Check sheet for the drawn part. Datum: minimum x, y, z corner. Units: mm. A direction names the side the tool comes from. Round coordinates to 2 decimals unless told otherwise and drop trailing zeros. Loops run counter-clockwise (first coordinate to the right, second up) from the corner with the lowest first, then second, coordinate; pieces in that order, holes last. Notation, with made-up numbers: (67.25, 14) - (125.25, 14) arc R17 ccw to (125.25, 30) - close; hole circle Ø11 at (50, 22.5). An arc over 180 degrees is marked (long way). Use CSV: the item, a comma, the result in double quotes.
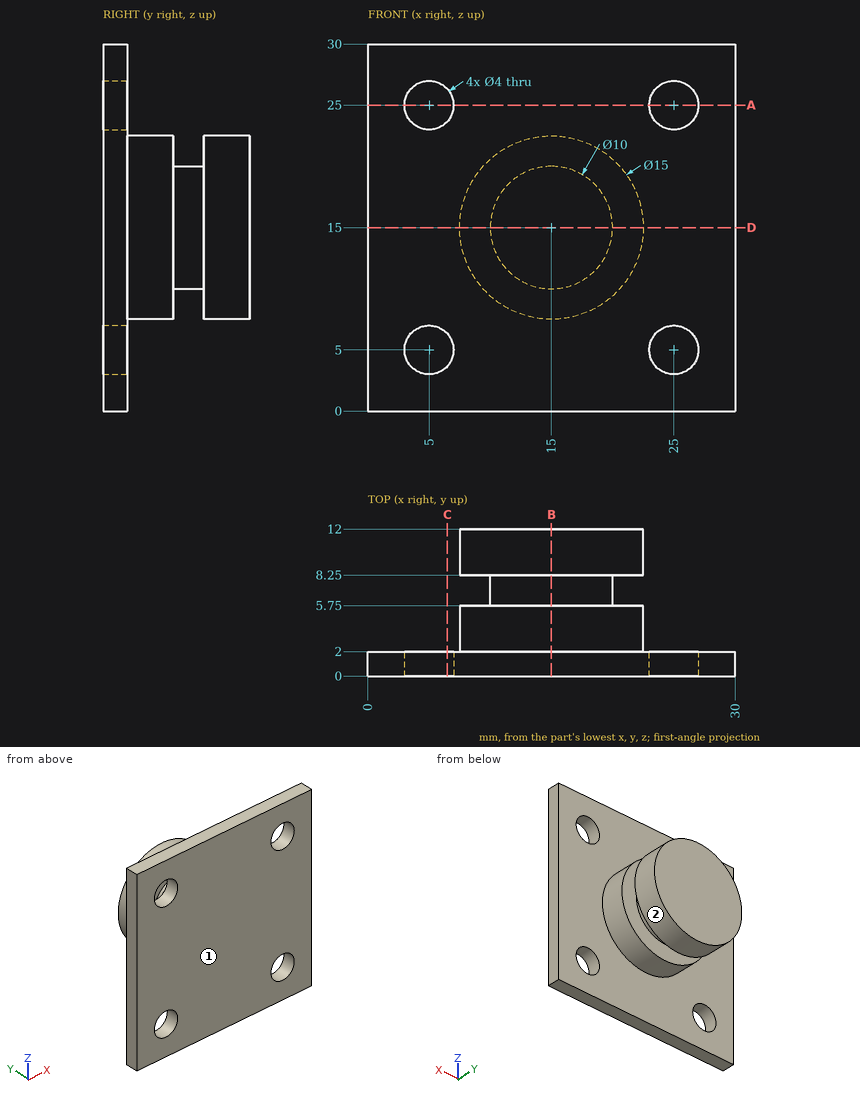
1) Cross-section at A-A, the plane z = 25. Record the cut outline in (x, y).
Returned:
outline,"(0, 0) - (3, 0) - (3, 2) - (0, 2) - close; (7, 0) - (23, 0) - (23, 2) - (7, 2) - close; (27, 0) - (30, 0) - (30, 2) - (27, 2) - close"
2) Cross-section at D-D, the plane z = 15. Record the cut outline in (x, y).
Returned:
outline,"(0, 0) - (30, 0) - (30, 2) - (22.5, 2) - (22.5, 5.75) - (20, 5.75) - (20, 8.25) - (22.5, 8.25) - (22.5, 12) - (7.5, 12) - (7.5, 8.25) - (10, 8.25) - (10, 5.75) - (7.5, 5.75) - (7.5, 2) - (0, 2) - close"
3) Thickness scan on probe 1 along X at (y, z) = (0.7, 5); probe 2 along Y at (x, z) = (14.25, 9.75). Record the ranges inside material, lowest first. Write a range as [from, to].
Returned:
probe 1,"x = [0, 3], [7, 23], [27, 30]"
probe 2,"y = [0, 5.75], [8.25, 12]"
4) Access from +Z, -Z, +X, -X, +Y, -Y to the whole of each face (thin tool, end or side, straight path). Record for the marked faces 1 and 2.
Returned:
face 1,"+Z, -Z, +X, -X, -Y"
face 2,"+Y"
5) Cross-section at B-B, the plane x = 15. Record the cut outline in (y, z).
Returned:
outline,"(0, 0) - (2, 0) - (2, 7.5) - (5.75, 7.5) - (5.75, 10) - (8.25, 10) - (8.25, 7.5) - (12, 7.5) - (12, 22.5) - (8.25, 22.5) - (8.25, 20) - (5.75, 20) - (5.75, 22.5) - (2, 22.5) - (2, 30) - (0, 30) - close"
6) Cross-section at C-C, the plane x = 6.5. Record the cut outline in (y, z), then the cut area to 3 significant figures.
Returned:
outline,"(0, 0) - (2, 0) - (2, 3.68) - (0, 3.68) - close; (0, 6.32) - (2, 6.32) - (2, 23.68) - (0, 23.68) - close; (0, 26.32) - (2, 26.32) - (2, 30) - (0, 30) - close"
area,"49.4 mm²"
7) Gauge pin test, flat ends, axial feed: pin 1 Ø3 at (x, z) = (25, 25) entering from +Y; pin 2 Ø4 at (x, z) = (19.5, 26.5) entering from +Y; pin 3 Ø1 at (y, z) = (10, 15) entering from -X; pin 4 Ø1 at (y, z) = (8.5, 20) entering from -X. Record the tip position at first contact, or that the pin passes through.
Returned:
pin 1,"passes through"
pin 2,"stops at y = 2"
pin 3,"stops at x = 7.5"
pin 4,"stops at x = 9"
